from build123d import *

# Parameters (mm, degrees)
SKETCH1_W           = 57.5
SKETCH1_H           = 15
SKETCH1_W_2         = 4
SKETCH1_H_2         = 7
BOSS_EXTRUDE1_DEPTH = 6.75
SKETCH2_R           = 1.875
CUT_EXTRUDE1_DEPTH  = 60.806458681


with BuildPart() as part:
    # Sketch1 → Boss-Extrude1 (new body)
    with BuildSketch(Plane(origin=(0, 0, 0), x_dir=(1, 0, 0), z_dir=(0, 1, 0))):
        with Locations((28.75, 7.5)):
            Rectangle(SKETCH1_W, SKETCH1_H)
        with Locations((19.75, 7.5)):
            Rectangle(SKETCH1_W_2, SKETCH1_H_2, mode=Mode.SUBTRACT)
        with Locations((25.75, 7.5)):
            Rectangle(SKETCH1_W_2, SKETCH1_H_2, mode=Mode.SUBTRACT)
        with Locations((31.75, 7.5)):
            Rectangle(SKETCH1_W_2, SKETCH1_H_2, mode=Mode.SUBTRACT)
        with Locations((37.75, 7.5)):
            Rectangle(SKETCH1_W_2, SKETCH1_H_2, mode=Mode.SUBTRACT)
    extrude(amount=BOSS_EXTRUDE1_DEPTH)

    # Sketch2 → Cut-Extrude1 (cut, through all)
    with BuildSketch(Plane(origin=(0, 0, -15), x_dir=(-1, 0, 0), z_dir=(0, 0, -1))):
        with Locations((-53.75, 3.375)):
            Circle(SKETCH2_R)
        with Locations((-3.75, 3.375)):
            Circle(SKETCH2_R)
    extrude(amount=-CUT_EXTRUDE1_DEPTH, mode=Mode.SUBTRACT)


solid = part.part
Part model, mm, in its own coordinate system. A direction names the side the tool comes from. Coordinates: 2 decimals unless noted, no trailing zeros. Write each loop counter-clockwise with the first axis right and the second up, starting at its lowest first coordinate (ties: lowest second). Pieces come first, ordered by that corner, then holes. Notation, with made-up numbers: M 50,73 L 109,73 A20 cw 109,110 Z; hole C 80,-22 d9. An arc over 180 degrees is marked long. Return JSON: item names as keys, results as strings.
1. Saw through at D-D, the plane z = -13. Write the cut outline in (x, y) (3 decimals).
Determined:
{"outline": "M 0,0 L 57.5,0 L 57.5,6.75 L 0,6.75 Z; hole C 3.75,3.375 d3.75; hole C 53.75,3.375 d3.75"}
2. Saw through at B-B, the plane z = -6. Write the cut outline in (x, y) (3 decimals).
Determined:
{"outline": "M 0,0 L 17.75,0 L 17.75,6.75 L 0,6.75 Z; M 21.75,0 L 23.75,0 L 23.75,6.75 L 21.75,6.75 Z; M 27.75,0 L 29.75,0 L 29.75,6.75 L 27.75,6.75 Z; M 33.75,0 L 35.75,0 L 35.75,6.75 L 33.75,6.75 Z; M 39.75,0 L 57.5,0 L 57.5,6.75 L 39.75,6.75 Z; hole C 3.75,3.375 d3.75; hole C 53.75,3.375 d3.75"}
3. Saw through at A-A, the plane x = 3.75. Write the cut outline in (y, z), then the cut area to 3 significant figures.
Determined:
{"outline": "M 0,-15 L 1.5,-15 L 1.5,0 L 0,0 Z; M 5.25,-15 L 6.75,-15 L 6.75,0 L 5.25,0 Z", "area": "45.0 mm²"}
4. Probe L1, parallel to X at y = 3.5, z = -0.75; L2, parallel to X at y = 6, z = -8.5; L3, parallel to Y at x = 3.75, z = -8.5. List the from-to ranges inside material, lowest first.
Determined:
{"L1": "0 to 1.88, 5.62 to 51.88, 55.62 to 57.5", "L2": "0 to 17.75, 21.75 to 23.75, 27.75 to 29.75, 33.75 to 35.75, 39.75 to 57.5", "L3": "0 to 1.5, 5.25 to 6.75"}
5. 3-axis set-ups, long thin cutter, end or side, ignore diameter. For faces 4 (the face through (0, 3, -7)), 5 (the face through (29.75, 3, -7)): which of +Z, -Z, +X, -X, +Y, -Y reach the whole face in a straight line?
Determined:
{"face 4": "+Z, -Z, -X, +Y, -Y", "face 5": "+Y, -Y"}
6. Saw through at C-C, the plane x = 26. Write the cut outline in (y, z).
Determined:
{"outline": "M 0,-15 L 6.75,-15 L 6.75,-11 L 0,-11 Z; M 0,-4 L 6.75,-4 L 6.75,0 L 0,0 Z"}
7. Pull direction Y, two halves, no side cores. Call faces 1 (the face through (35.75, 3, -7)), 2 (the face through (5.238, 2.234, -7.605)), 3 (the face through (28, 6.75, -8)): pulls with the +Y half, pulls with the -Y half, needs draft (parallel to the pull), parting line crosses it, or undercut.
Determined:
{"face 1": "needs draft", "face 2": "undercut", "face 3": "pulls with the +Y half"}
